Source: CAD feature listing. Evaluate the final solid. Frame: model axes, mm. A direction names the side the tool comes from. Give positions to 0.01 mm unless a question says otherwise; leave off trailing zeros. Order: outer loops, then holes, each group sorted by start corner. A loop starts at its lowest first (then second) coordinate and runs counter-clockwise, first axis right, second up. Notation, with made-up numbers: M 47.5,1 L 56.5,1 A23 cw 56.5,34 Z; hole C 60,-35.5 d4. An arc over 180 degrees is marked long. Answer as a JSON object with one key per item and string values. Group by question number.
1. Section query C-C (y = 3.5). Output: boundary loops of the cut face in (x, z).
2. Pull-direction query (X, two-part tool) for faces 3 (the cylindrical face through (23.166, 4.106, 1.517)), 4 (the flat face through (-19.4, 1, 9.4)), 5 (the cylindrical face through (-32.9, 4.2, 30.7)); classes: +X half, -X half, draft (parallel to the pull), parting line (faces both ways), or undercut.
3. Set-up query: faces 1 (the cylindrical face through (-1.517, 4.106, 23.166)), 2 (the flat face through (-1, 7.3, 19)). Return all of +Z, -Z, +X, -X, +Y, -Y with unobstructed straight access to the full face (end or side cutting, diameter ignored); none if empty.
4. Section query D-D (z = -30). Output: boundary loops of the cut face in (x, y).
5. Pin query (flat end, axial travel): P1, Ø3, axis at x = -17, z = 10.5, coming from the +Y side; P2, Ø11, axis at x = 0, z = 30, coming from the -Y side; P3, Ø2, axis at x = -21.5, z = -30.5, coming from the -Y side; P4, Ø6, axis at x = -10, y = 2, coming from the -Z side. Return the tip coordinate at first contact, or that it passes through.
6. Section query A-A (x = 0). Output: boundary loops of the cut face in (y, z), plus the area to 3 significant figures.
7. Section query B-B (x = -24.5). Output: boundary loops of the cut face in (y, z), plus the area to 3 significant figures.
8. Material intervals for L1, parallel to Z at x = 0, y = 2.5; L2, parallel to X at y = 7, z = 2; L3, parallel to Z at x = -4, y = 5, sorted ascending. Write a range as [from, to].
from build123d import *

# Parameters (mm, degrees)
F_14_0_14_DURCHMESSER_BOHRUNG2_D = 14
KREISMUSTER2_COUNT               = 4
F_3_8_18_NPSM_GEWINDEBOHRUNG1_D  = 15.3162
SCHNITT_LINEAR_AUSTRAGEN1_DEPTH  = 6.3
F_5_3_5_3_DURCHMESSER_BOHRUNG1_D = 5.3


with BuildPart() as part:
    # Skizze1 → Rotation1 (revolve)
    with BuildSketch(Plane.XY):
        Polygon((15, 12), (0, 12), (0, 0), (20, 0), (21, 1), (45, 1), (45, 7.3), (18, 7.3), align=None)
    revolve(axis=Axis((0, 0, 0), (0, 1, 0)))

    # Ø14.0 (14) Durchmesser Bohrung2 (through all)
    with Locations(Plane(origin=(0, 7.3, 0), x_dir=(1, 0, 0), z_dir=(0, 1, 0))):
        with Locations((0, 30)):
            f_14_0_14_durchmesser_bohrung2 = Hole(F_14_0_14_DURCHMESSER_BOHRUNG2_D / 2)

    # Kreismuster2: Ø14.0 (14) Durchmesser Bohrung2 ×4 about axis
    kreismuster2_axis = Axis((0, 0, 0), (0, 1, 0))
    for i in range(1, KREISMUSTER2_COUNT):
        add(f_14_0_14_durchmesser_bohrung2.rotate(kreismuster2_axis, i * 360 / KREISMUSTER2_COUNT), mode=Mode.SUBTRACT)

    # 3/8-18 NPSM Gewindebohrung1 (through all)
    with Locations(Plane(origin=(0, 12, 0), x_dir=(1, 0, 0), z_dir=(0, 1, 0))):
        with Locations((0, 0)):
            Hole(F_3_8_18_NPSM_GEWINDEBOHRUNG1_D / 2)

    # Skizze16 → Schnitt-Linear austragen1 (cut)
    with BuildSketch(Plane(origin=(0, 7.3, 0), x_dir=(1, 0, 0), z_dir=(0, 1, 0))):
        with BuildLine():
            Line((44.933664947, 2.442489393), (2.442489393, 44.933664947))
            ThreePointArc((2.442489393, 44.933664947), (31.819805153, 31.819805153), (44.933664947, 2.442489393))
        make_face()
    extrude(amount=-SCHNITT_LINEAR_AUSTRAGEN1_DEPTH, mode=Mode.SUBTRACT)

    # Ø5.3 (5.3) Durchmesser Bohrung1 (through all)
    with Locations(Plane(origin=(0, 7.3, 0), x_dir=(1, 0, 0), z_dir=(0, 1, 0))):
        with Locations((13.25528115, 19.978737566)):
            Hole(F_5_3_5_3_DURCHMESSER_BOHRUNG1_D / 2)


solid = part.part
Answer sheet:
{
 "1": {"outline": "M 2.44,-44.93 L 44.93,-2.44 A45 ccw long Z; hole C -30,0 d14; hole C 0,0 d15.32; hole C 0,-30 d14; hole C 0,30 d14; hole C 13.26,-19.98 d5.3; hole C 30,0 d14"},
 "2": {"face 3": "undercut", "face 4": "draft", "face 5": "parting line"},
 "3": {"face 1": "+Y, -Y", "face 2": "+Y"},
 "4": {"outline": "M -33.54,1 L -7,1 L -7,7.3 L -33.54,7.3 Z; M 7,1 L 17.38,1 L 17.38,7.3 L 7,7.3 Z"},
 "5": {"P1": "y = 7.3", "P2": "through", "P3": "y = 1", "P4": "z = -44.45"},
 "6": {"outline": "M 0,-20 L 1,-21 L 1,-23 L 7.3,-23 L 7.3,-18 L 12,-15 L 12,-7.66 L 0,-7.66 Z; M 0,7.66 L 12,7.66 L 12,15 L 7.3,18 L 7.3,23 L 1,23 L 1,21 L 0,20 Z; M 1,-45 L 7.3,-45 L 7.3,-37 L 1,-37 Z; M 1,37 L 7.3,37 L 7.3,45 L 1,45 Z", "area": "403 mm^2"},
 "7": {"outline": "M 1,-37.75 L 7.3,-37.75 L 7.3,-4.33 L 1,-4.33 Z; M 1,4.33 L 7.3,4.33 L 7.3,37.75 L 1,37.75 Z", "area": "421 mm^2"},
 "8": {"L1": "[-45, -37], [-23, -7.66], [7.66, 23], [37, 45]", "L2": "[-44.96, -36.71], [-23.29, -7.39], [7.39, 23.29], [36.71, 44.96]", "L3": "[-44.82, -35.74], [-24.26, -6.53], [6.53, 24.26], [35.74, 44.82]"}
}
